Can you work these out from the model? Positions are in its coordinate system, mm. Round coordinates to 2 decimals unless told otherwise and drop trailing zeros. Write each loop counter-clockwise with the first axis right and the second up, starting at its lowest first coordinate (ties: lowest second). Pieces come first, ordered by that corner, then holes.
Q1. If we section it at A-A (y = -1.4): Please give me the cut outline in (x, z), plus the area to 3 significant figures.
Q2. If we section it at D-D (z = 17.5): Please give me the cut outline in (x, y).
Q3. If we section it at C-C (x = -25.5): Please give me the cut outline in (y, z).
Q4. If we section it at B-B (x = 54.5): Please give me the cut outline in (y, z).
Q5. I'm going to push flat-ended pins straight in: pin 1 Ø1.1 at (x, y) = (-42, -1.5) entering from -Z; pin 2 Ø1.1 at (x, y) = (48.5, -1) entering from -Z; pin 3 Ø1.1 at (x, y) = (-39, -1.5) entering from +Z. Where does each tip first touch, or does it pass through?
Q6. Please list where these lines run through material, in increasing order: line 1 along Z through (x, y) = (51.5, -0.2); line 2 along Z through (x, y) = (-40.5, -0.25); line 3 along X through (y, z) = (-0.85, -0.5).
from build123d import *

# Parameters (mm, degrees)
F2_DEPTH  = 2.286
F4_DEPTH  = 2.286
F5_R      = 2.0707192567
F7_R      = 8.2702748321
F8_R      = 2.754363365
F9_DEPTH  = 25.4
F11_DEPTH = 0.127
F13_DEPTH = 25.4


with BuildPart() as f2:
    # F0 (on Front) → F2 (new body)
    with BuildSketch(Plane.XZ):
        with BuildLine():
            Line((-50.8, -12.7), (35.2199618575, -12.7))
            ThreePointArc((35.2199618575, -12.7), (30.6995624794, 0), (35.2199618575, 12.7))
            Line((35.2199618575, 12.7), (-50.8, 12.7))
            Line((-50.8, 12.7), (-50.8, -12.7))
        make_face()
        with BuildLine():
            Line((41.0022673368, -14.1657050699), (41.0022673368, -12.7))
            Line((41.0022673368, -12.7), (35.2199618575, -12.7))
            ThreePointArc((35.2199618575, -12.7), (57.5402524162, -18.9366466379), (70.9004375206, 0))
            ThreePointArc((70.9004375206, 0), (57.5402524162, 18.9366466379), (35.2199618575, 12.7))
            Line((35.2199618575, 12.7), (41.0022673368, 12.7))
            Line((41.0022673368, 12.7), (41.0022673368, 14.1657050699))
            Line((41.0022673368, 14.1657050699), (60.5977326632, 14.1657050699))
            Line((60.5977326632, 14.1657050699), (60.5977326632, -14.1657050699))
            Line((60.5977326632, -14.1657050699), (41.0022673368, -14.1657050699))
        make_face()
        with BuildLine():
            Line((35.2199618575, -12.7), (41.0022673368, -12.7))
            Line((41.0022673368, -12.7), (41.0022673368, 12.7))
            Line((41.0022673368, 12.7), (35.2199618575, 12.7))
            ThreePointArc((35.2199618575, 12.7), (30.6995624794, 0), (35.2199618575, -12.7))
        make_face()
    extrude(amount=F2_DEPTH)

    # F3 (on face) → F4 (join)
    with BuildSketch(Plane.XZ.offset(2.286)):
        with BuildLine():
            Line((41.0022673368, 8.3944918588), (41.0022673368, -8.3944918588))
            ThreePointArc((41.0022673368, -8.3944918588), (49.3967591956, 0), (41.0022673368, 8.3944918588))
        make_face()
    extrude(amount=-F4_DEPTH)

    # F5
    f5_edges = [f2.edges().sort_by_distance(p)[0] for p in [
        (41.002267, -1.143, 14.165705),
        (41.002267, -1.143, -14.165705),
    ]]
    fillet(f5_edges, radius=F5_R)

    # F7
    f7_edges = [f2.edges().sort_by_distance(p)[0] for p in [
        (60.597733, -1.143, -14.165705),
        (60.597733, -1.143, 14.165705),
    ]]
    fillet(f7_edges, radius=F7_R)

    # F8 (on face) → F9 (cut)
    with BuildSketch(Plane.XZ.offset(2.286)):
        with Locations((66.192291677, 0)):
            Circle(F8_R)
    extrude(amount=-F9_DEPTH, mode=Mode.SUBTRACT)

    # F10 (on face) → F11 (cut)
    with BuildSketch(Plane(origin=(0, 0, 0), x_dir=(-1, 0, 0), z_dir=(0, 1, 0))):
        with BuildLine():
            ThreePointArc((-45.3273802996, 7.1945042516), (-49.3967591956, 0), (-45.3273802996, -7.1945042516))
            Line((-45.3273802996, -7.1945042516), (-45.3273802996, 7.1945042516))
        make_face()
    extrude(amount=-F11_DEPTH, mode=Mode.SUBTRACT)

    # F12 (on face) → F13 (cut)
    with BuildSketch(Plane(origin=(0, 0, 0), x_dir=(-1, 0, 0), z_dir=(0, 1, 0))):
        Polygon((44.0986434706, 6.1829173937), (36.9592254273, 6.1829173937), (33.3895164056, 0), (36.9592254273, -6.1829173937), (44.0986434706, -6.1829173937), (47.6683524923, 0), align=None)
    extrude(amount=-F13_DEPTH, mode=Mode.SUBTRACT)


solid = f2.part
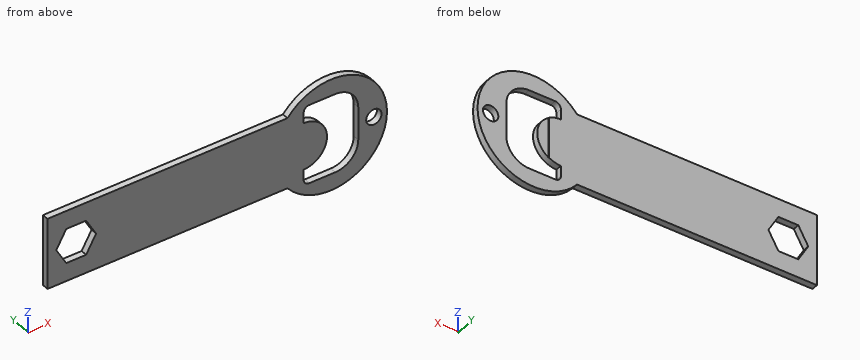
A:
1. outline: (-50.8, -12.7) - (35.22, -12.7) arc R20.1 ccw (long way) to (35.22, 12.7) - (-50.8, 12.7) - close; hole (-47.67, 0) - (-44.1, -6.18) - (-36.96, -6.18) - (-33.39, 0) - (-36.96, 6.18) - (-44.1, 6.18) - close; hole (41, -12.09) arc R2.07 ccw to (43.07, -14.17) - (52.33, -14.17) arc R8.27 ccw to (60.6, -5.9) - (60.6, 5.9) arc R8.27 ccw to (52.33, 14.17) - (43.07, 14.17) arc R2.07 ccw to (41, 12.09) - (41, 8.39) arc R8.39 cw to (41, -8.39) - close; hole circle Ø5.51 at (66.19, 0)
1. area: 2,810 mm2
2. outline: (40.91, -2.29) - (60.69, -2.29) - (60.69, 0) - (40.91, 0) - close
3. outline: (-2.29, -12.7) - (0, -12.7) - (0, 12.7) - (-2.29, 12.7) - close
4. outline: (-2.29, -19.76) - (0, -19.76) - (0, -13.88) - (-2.29, -13.88) - close; (-2.29, 13.88) - (0, 13.88) - (0, 19.76) - (-2.29, 19.76) - close
5. pin 1: stops at z = -12.7
5. pin 2: stops at z = -20.02
5. pin 3: stops at z = 12.7
6. line 1: z = -20.09 to -14.17, 14.17 to 20.09
6. line 2: z = -12.7 to -6.18, 6.18 to 12.7
6. line 3: x = -50.8 to -47.38, -33.68 to 49.38, 60.6 to 63.48, 68.9 to 70.89
